```python
from build123d import *

# Parameters (mm, degrees)
SKETCH_1_W          = 22.033021484
SKETCH_1_H          = 26.449100754
SKETCH_1_R          = 0.925
EXTRUDE_1_DEPTH     = 5
SKETCH_1_3_W        = 22.033021484
SKETCH_1_3_H        = 5
EXTRUDE_2_DEPTH     = 35
SKETCH_3_R          = 0.925
CUT_EXTRUDE_1_DEPTH = 25


with BuildPart() as part:
    # Sketch 1 → Extrude 1 (new body)
    with BuildSketch(Plane(origin=(0, 0, 0), x_dir=(1, 0, 0), z_dir=(0, 1, 0))):
        Rectangle(SKETCH_1_W, SKETCH_1_H)
        with Locations(Location((7.25, 0, 0), (0, 0, 270))):
            Circle(SKETCH_1_R, mode=Mode.SUBTRACT)
        with Locations(Location((7.25, 3.25, 0), (0, 0, 270))):
            Circle(SKETCH_1_R, mode=Mode.SUBTRACT)
        with Locations(Location((-3.5, -7.25, 0), (0, 0, 270))):
            Circle(SKETCH_1_R, mode=Mode.SUBTRACT)
        with Locations(Location((3.5, 7.25, 0), (0, 0, 270))):
            Circle(SKETCH_1_R, mode=Mode.SUBTRACT)
        with Locations(Location((-3.5, 7.25, 0), (0, 0, 270))):
            Circle(SKETCH_1_R, mode=Mode.SUBTRACT)
        with Locations(Location((0, 7.25, 0), (0, 0, 270))):
            Circle(SKETCH_1_R, mode=Mode.SUBTRACT)
        with Locations(Location((3.5, -7.25, 0), (0, 0, 270))):
            Circle(SKETCH_1_R, mode=Mode.SUBTRACT)
        with Locations(Location((0, -7.25, 0), (0, 0, 270))):
            Circle(SKETCH_1_R, mode=Mode.SUBTRACT)
        with Locations(Location((-7.25, 0, 0), (0, 0, 270))):
            Circle(SKETCH_1_R, mode=Mode.SUBTRACT)
        with Locations(Location((-7.25, -3.25, 0), (0, 0, 270))):
            Circle(SKETCH_1_R, mode=Mode.SUBTRACT)
        with Locations(Location((-7.25, 3.25, 0), (0, 0, 270))):
            Circle(SKETCH_1_R, mode=Mode.SUBTRACT)
        with Locations(Location((7.25, -3.25, 0), (0, 0, 270))):
            Circle(SKETCH_1_R, mode=Mode.SUBTRACT)
    extrude(amount=-EXTRUDE_1_DEPTH)

    # Sketch 1_3 → Extrude 2 (add)
    with BuildSketch(Plane(origin=(0, 0, 0), x_dir=(1, 0, 0), z_dir=(0, 1, 0))):
        with Locations((0, 15.724550377)):
            Rectangle(SKETCH_1_3_W, SKETCH_1_3_H)
    extrude(amount=-EXTRUDE_2_DEPTH)

    # Sketch 3 → Cut-Extrude 1 (cut)
    with BuildSketch(Plane.XY.offset(-13.224550377)):
        with Locations((0, -13)):
            Circle(SKETCH_3_R)
        with Locations((-3.5, -13)):
            Circle(SKETCH_3_R)
        with Locations((3.5, -13)):
            Circle(SKETCH_3_R)
        with Locations((3.5, -27.5)):
            Circle(SKETCH_3_R)
        with Locations((0, -27.5)):
            Circle(SKETCH_3_R)
        with Locations((-3.5, -27.5)):
            Circle(SKETCH_3_R)
        with Locations((-7.5, -20.25)):
            Circle(SKETCH_3_R)
        with Locations((-7.5, -16.75)):
            Circle(SKETCH_3_R)
        with Locations((-7.5, -23.75)):
            Circle(SKETCH_3_R)
        with Locations((7.5, -16.75)):
            Circle(SKETCH_3_R)
        with Locations((7.5, -20.25)):
            Circle(SKETCH_3_R)
        with Locations((7.5, -23.75)):
            Circle(SKETCH_3_R)
    extrude(amount=-CUT_EXTRUDE_1_DEPTH, mode=Mode.SUBTRACT)


solid = part.part
```
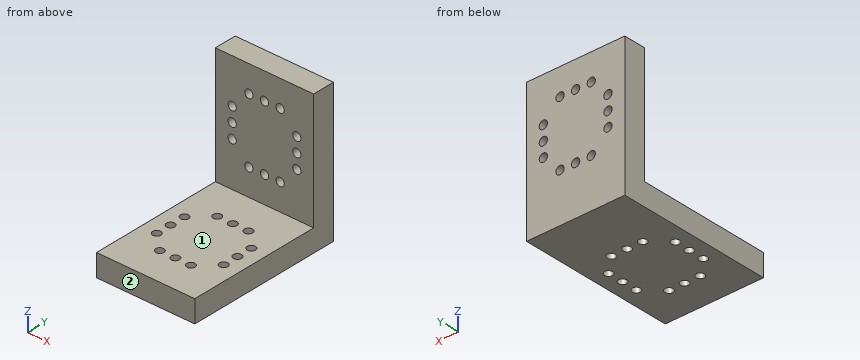
Verification items for the finished model (mm, model axes). Face numbers are marked on the shaded views. A direction names the side the tool comes from. Coordinates: 2 decimals unless noted, no trailing zeros. Loops run counter-clockwise (first coordinate to the right, second up) from the corner with the lowest first, then second, coordinate; pieces in that order, holes last. Notation, with made-up numbers: (-19, 30) -> (-12, 30) arc R26 cw to (-12, 44) -> close; hole circle Ø5 at (87, 35.25). An arc over 180 degrees is marked (long way). Answer in a Markdown table with one row per item. Add a question column.
1. Section check C-C, the plane y = -13. Enter the section's corners in (x, z) (3 decimals).
2. Material ranges on probe 1 along Y at (x, z) = (3.5, -16.55) (3 decimals); probe 2 along Z at (x, y) = (-4, -3); probe 3 along X at (y, z) = (-3, 7), recorded low to high. Write a range as [from, to].
3. Section check D-D, the plane y = -23.75. Enter the section's corners in (x, z) (3 decimals).
4. Depth check by flat-ended pin: P1, Ø1.5, axis at x = -7.25, z = 0, coming from the +Y side; P2, Ø10, axis at x = -1, y = -13, coming from the +Z side; P3, Ø12, axis at x = -5.5, z = -3, coming from the -Y side. Enter the tip coordinate at first touch or a pass-through.
5. Access from +Z, -Z, +X, -X, +Y, -Y to the whole of each face (thin tool, end or side, straight path). Record for the marked faces 1 and 2.
6. Section check B-B, the plane x = 0. Enter the section's corners in (y, z) (3 decimals), then the cut area to 3 significant figures.
7. Section check A-A, the plane z = 7.25. Enter the section's corners in (x, y) (3 decimals).
Derived:
| question | item | result |
|---|---|---|
| 1 | outline | (-11.017, -18.225) -> (-4.425, -18.225) -> (-4.425, -13.225) -> (-11.017, -13.225) -> close; (-2.575, -18.225) -> (-0.925, -18.225) -> (-0.925, -13.225) -> (-2.575, -13.225) -> close; (0.925, -18.225) -> (2.575, -18.225) -> (2.575, -13.225) -> (0.925, -13.225) -> close; (4.425, -18.225) -> (11.017, -18.225) -> (11.017, -13.225) -> (4.425, -13.225) -> close |
| 2 | probe 1 | y = [-35, -28.425], [-26.575, -13.925], [-12.075, 0] |
| 2 | probe 2 | z = [-18.22, -8.03], [-6.47, 6.47], [8.03, 13.22] |
| 2 | probe 3 | x = [-11.02, -4.39], [-2.61, -0.89], [0.89, 2.61], [4.39, 11.02] |
| 3 | outline | (-11.017, -18.225) -> (-8.425, -18.225) -> (-8.425, -13.225) -> (-11.017, -13.225) -> close; (-6.575, -18.225) -> (6.575, -18.225) -> (6.575, -13.225) -> (-6.575, -13.225) -> close; (8.425, -18.225) -> (11.017, -18.225) -> (11.017, -13.225) -> (8.425, -13.225) -> close |
| 4 | P1 | passes through |
| 4 | P2 | stops at z = -13.22 |
| 4 | P3 | stops at y = -5 |
| 5 | face 1 | +Z, +X, -X, -Y |
| 5 | face 2 | +Z, -Z, +X, -X, -Y |
| 6 | outline | (-35, -18.225) -> (-28.425, -18.225) -> (-28.425, -13.225) -> (-35, -13.225) -> close; (-26.575, -18.225) -> (-13.925, -18.225) -> (-13.925, -13.225) -> (-26.575, -13.225) -> close; (-12.075, -18.225) -> (0, -18.225) -> (0, -8.175) -> (-5, -8.175) -> (-5, -13.225) -> (-12.075, -13.225) -> close; (-5, -6.325) -> (0, -6.325) -> (0, 6.325) -> (-5, 6.325) -> close; (-5, 8.175) -> (0, 8.175) -> (0, 13.225) -> (-5, 13.225) -> close |
| 6 | area | 270 mm² |
| 7 | outline | (-11.017, -5) -> (-4.425, -5) -> (-4.425, 0) -> (-11.017, 0) -> close; (-2.575, -5) -> (-0.925, -5) -> (-0.925, 0) -> (-2.575, 0) -> close; (0.925, -5) -> (2.575, -5) -> (2.575, 0) -> (0.925, 0) -> close; (4.425, -5) -> (11.017, -5) -> (11.017, 0) -> (4.425, 0) -> close |
